Autodesk Inventor part; units mm, degrees
ref_plane "YZ Plane" through (0, 0, 0) normal (1, 0, 0) x (0, 1, 0)
ref_plane "XZ Plane" through (0, 0, 0) normal (0, 1, 0) x (-1, 0, 0)
ref_plane "XY Plane" through (0, 0, 0) normal (0, 0, 1) x (1, 0, 0)
sketch "Sketch1" plane through (0, 0, 0) normal (0, 1, 0) x (-1, 0, 0)
  line L0 (375, 250) -> (-375, 250)
  line L1 (-375, 250) -> (-375, -250)
  line L2 (-375, -250) -> (375, -250)
  line L3 (375, -250) -> (375, 250)
  line L4 (375, 250) -> (-375, -250) construction
  line L5 (-375, 250) -> (375, -250) construction
  point P0 (0, 0)
  dimension "d0" = 750
  dimension "d1" = 500
extrude "Extrusion1" add sketch "Sketch1" along normal blind 100
sketch "Sketch2" plane through (0, 100, 0) normal (0, 1, 0) x (1, 0, 0)
  line L0 (-150, -200) -> (150, -200)
  line L1 (200, -150) -> (200, 150)
  line L2 (150, 200) -> (-150, 200)
  line L3 (-200, 150) -> (-200, -150)
  line L4 (-200, -200) -> (200, 200) construction
  line L5 (200, -200) -> (-200, 200) construction
  arc A0 (-200, -150) -> (-150, -200) centre (-150, -150) ccw
  arc A1 (-150, 200) -> (-200, 150) centre (-150, 150) ccw
  arc A2 (150, -200) -> (200, -150) centre (150, -150) ccw
  arc A3 (200, 150) -> (150, 200) centre (150, 150) ccw
  point P0 (0, 0)
  dimension "d4" = 400
  dimension "d5" = 400
  dimension "d6" = 50
  dimension "d7" = 50
  dimension "d8" = 50
extrude "Extrusion2" cut sketch "Sketch2" against normal blind 75
fillet "Fillet1" radius 25 12 edges at (375, 50, -250) (375, 0, 0) (375, 100, 0) (375, 50, 250) (0, 100, 250) (0, 100, -250) (-375, 100, 0) (0, 0, -250) (-375, 50, -250) (-375, 0, 0) (-375, 50, 250) (0, 0, 250)
sketch "Sketch3" plane through (0, 0, 0) normal (0, -1, 0) x (1, 0, 0)
  line L0 (300, -175) -> (-300, 175) construction
  line L1 (-300, -175) -> (300, 175) construction
  circle A0 centre (-300, -175) radius 25
  circle A1 centre (-300, 175) radius 25
  circle A2 centre (0, -175) radius 25
  circle A3 centre (0, 175) radius 25
  circle A4 centre (300, -175) radius 25
  circle A5 centre (300, 175) radius 25
  point P0 (0, 0)
  dimension "d12" = 600
  dimension "d13" = 350
  dimension "d14" = 50
  dimension "d15" = 50
  dimension "d16" = 50
  dimension "d17" = 50
  dimension "d18" = 50
  dimension "d19" = 50
extrude "Extrusion3" cut sketch "Sketch3" against normal blind 10
sketch "Sketch4" plane through (0, 25, 0) normal (0, 1, 0) x (1, 0, 0)
  circle A0 centre (-150, 150) radius 22.5
  arc A1 (-150, 200) -> (-200, 150) centre (-150, 150) ccw
  circle A2 centre (150, 150) radius 22.5
  circle A3 centre (150, -150) radius 22.5
  circle A4 centre (-150, -150) radius 22.5
  arc A5 (200, 150) -> (150, 200) centre (150, 150) ccw
  arc A6 (150, -200) -> (200, -150) centre (150, -150) ccw
  arc A7 (-200, -150) -> (-150, -200) centre (-150, -150) ccw
  point P0 (0, 0)
  dimension "d22" = 45
  dimension "d23" = 45
  dimension "d24" = 45
  dimension "d25" = 45
extrude "Extrusion4" add sketch "Sketch4" along normal blind 25
properties part number "WHEEL_BASE" material "Stainless Steel"
Input: part model. Units: mm. Frame: model coordinates. A direction names the side the tool comes from. Give positions to 0.01 mm unless a question says otherwise; leave off trailing zeros. Write each loop counter-clockwise with the first axis right and the second up, starting at its lowest first coordinate (ties: lowest second). Pieces come first, ordered by that corner, then holes.
Q1. Section C-C, the plane z = -39. Output: boundary loops of the cut face in (x, y), plus the area to 3 significant figures.
Q2. Section B-B, the plane x = -69.5. Output: boundary loops of the cut face in (y, z).
Q3. First-contact query: P1, Ø6, axis at x = 60, z = -146.5, coming from the +Y side; P2, Ø1.5, axis at x = -118, y = 85, coming from the -Z side; P3, Ø13.5, axis at x = 141, z = -161, coming from the +Y side. Flat tips, straight axial feed; report the tip coordinate or a pass-through.
Q4. Material intervals for probe 1 along Z at (x, y) = (300, 2.75); probe 2 along Z at (x, y) = (297, 8); probe 3 along Y at (x, z) = (139.5, -66), sorted ascending.
Q5. Set-up query: faces 1 (the face through (-150, 50, 150)), 2 (the face through (323.846, 4.93, 182.509)), 3 (the face through (5, 100, 203)). Return all of +Z, -Z, +X, -X, +Y, -Y with unobstructed straight access to the full face (end or side cutting, diameter ignored); none if empty.
Q6. Section D-D, the plane y = 92. Output: boundary loops of the cut face in (x, z).
Q7. Pull-direction query (Z, two-part tool) for faces 4 (the face through (-4.9, 92.871, -242.482)), 5 (the face through (367.871, 7.518, -3.15)), 6 (the face through (-137.9, 37.33, 168.97)); classes: pulls with the +Z half, pulls with the -Z half, needs draft (parallel to the pull), parting line crosses it, or undercut.
Q8. Section A-A, the plane y = 41.5. Output: boundary loops of the cut face in (x, z), plus the area to 3 significant figures.
Filled in:
1. outline: (-375, 25) arc R25 ccw to (-350, 0) - (350, 0) arc R25 ccw to (375, 25) - (375, 75) arc R25 ccw to (350, 100) - (200, 100) - (200, 25) - (-200, 25) - (-200, 100) - (-350, 100) arc R25 ccw to (-375, 75) - close
1. area: 44,500 mm2
2. outline: (0, -225) arc R25 ccw to (25, -250) - (75, -250) arc R25 ccw to (100, -225) - (100, -200) - (25, -200) - (25, 200) - (100, 200) - (100, 225) arc R25 ccw to (75, 250) - (25, 250) arc R25 ccw to (0, 225) - close
3. P1: stops at y = 25
3. P2: stops at z = -248.23
3. P3: stops at y = 50
4. probe 1: z = -236.4 to -200, -150 to 150, 200 to 236.4
4. probe 2: z = -243.33 to -199.82, -150.18 to 150.18, 199.82 to 243.33
4. probe 3: y = 0 to 25
5. face 1: +Y
5. face 2: -Y
5. face 3: +Z, -Z, +X, -X, +Y
6. outline: (-368.33, -225) arc R18.33 ccw to (-350, -243.33) - (350, -243.33) arc R18.33 ccw to (368.33, -225) - (368.33, 225) arc R18.33 ccw to (350, 243.33) - (-350, 243.33) arc R18.33 ccw to (-368.33, 225) - close; hole (-200, -150) arc R50 ccw to (-150, -200) - (150, -200) arc R50 ccw to (200, -150) - (200, 150) arc R50 ccw to (150, 200) - (-150, 200) arc R50 ccw to (-200, 150) - close
7. face 4: pulls with the -Z half
7. face 5: needs draft
7. face 6: undercut
8. outline: (-375, -225) arc R25 ccw to (-350, -250) - (350, -250) arc R25 ccw to (375, -225) - (375, 225) arc R25 ccw to (350, 250) - (-350, 250) arc R25 ccw to (-375, 225) - close; circle Ø45 at (-150, -150); circle Ø45 at (-150, 150); circle Ø45 at (150, -150); circle Ø45 at (150, 150); hole (-200, -150) arc R50 ccw to (-150, -200) - (150, -200) arc R50 ccw to (200, -150) - (200, 150) arc R50 ccw to (150, 200) - (-150, 200) arc R50 ccw to (-200, 150) - close
8. area: 223,000 mm2
